Read the model definition and answer for the solid it produces. Units are mm, in the model's axes. Face numbers are marked on the shaded views. A direction names the side the tool comes from. Round coordinates to 2 decimals unless told otherwise and drop trailing zeros. Write each loop counter-clockwise with the first axis right and the second up, starting at its lowest first coordinate (ties: lowest second). Pieces come first, ordered by that corner, then holes. Notation, with made-up numbers: (31.25, 76.25) - (80.25, 76.25) arc R7 cw to (80.25, 82.25) - close; hole circle Ø8 at (10.25, -12.75). An arc over 180 degrees is marked (long way). Use one line per item in the form item = value. Start each with the question number.
1) Each of these flat-tipped pins is pushed along its axis until it touches: pin 1 (3 mm diameter, centred on x = 5.5, z = 3.5, fed in from -Y); pin 2 (1 mm diameter, centred on x = 8, z = 7.5, fed in from +Y); pin 3 (2 mm diameter, centred on x = 3.5, z = 4, fed in from -Y); pin 4 (2 mm diameter, centred on x = -21, z = -14.5, fed in from +Y). Where does it stop, or does it pass through?
2) The part is cut by section D-D, the plane x = -22.5. Give the vertices of the cut face in (y, z), plus the area to 3 significant figures.
3) The part is cut by section A-A, the plane x = -7.5. Give the vertices of the cut face in (y, z), plus the area to 3 significant figures.
4) For a pull along X with two mould halves and no side action, classify the marked faces 1, 2 and 3 as released by +X, released by -X, zero draft, split by the parting line, or undercut.
5) The part is cut by section B-B, the plane y = -1.5. Give the vertices of the cut face in (x, z).
6) The part is cut by section C-C, the plane z = 6. Give the vertices of the cut face in (x, y), plus the area to 3 significant figures.
7) Consider line 1 along X through (y, z) = (2.5, -17); line 2 along Z through (x, y) = (-17, -2.75); line 3 along Z through (x, y) = (-14, -0.75). Determine where each line is inside the solid, lowest interval first. Write a range as from..to.
8) For the marked faces 4, 5, 6, 7 and 8, determine the directions among +Z, -Z, +X, -X, +Y, -Y from which every point of the face is accessible in a straight line to the end or side of a thin tool.
from build123d import *

# Parameters (mm, degrees)
SKETCH_1_W          = 35
SKETCH_1_H          = 32
EXTRUDE_1_DEPTH     = 2
CUT_EXTRUDE_2_DEPTH = 2
SKETCH_3_W          = 35
SKETCH_3_H          = 4
EXTRUDE_2_DEPTH     = 4
SKETCH_4_W          = 35
SKETCH_4_H          = 2
CUT_EXTRUDE_3_DEPTH = 2
SKETCH_5_W          = 35
SKETCH_5_H          = 2
CUT_EXTRUDE_4_DEPTH = 2
SKETCH_6_W          = 5
SKETCH_6_H          = 4.571428571
SKETCH_6_H_2        = 4.571428572
EXTRUDE_3_DEPTH     = 2
SKETCH_7_W          = 25
SKETCH_7_H          = 4.571428572
SKETCH_7_H_2        = 4.571428571
CUT_EXTRUDE_5_DEPTH = 1
SKETCH_9_R          = 1
EXTRUDE_4_DEPTH     = 28
EXTRUDE_START       = -5
SKETCH_9_3_R        = 1
EXTRUDE_5_DEPTH     = 35


with BuildPart() as part:
    # 草图1 → 凸台-拉伸1 (new body)
    with BuildSketch(Plane(origin=(0, 0, 0), x_dir=(1, 0, 0), z_dir=(0, 1, 0))):
        with Locations((-7.669902913, 4.366504854)):
            Rectangle(SKETCH_1_W, SKETCH_1_H)
    extrude(amount=EXTRUDE_1_DEPTH)

    # 草图1<3> → 切除-拉伸2 (cut)
    with BuildSketch(Plane(origin=(0, 0, 0), x_dir=(1, 0, 0), z_dir=(0, 1, 0))):
        Polygon((-7.669902913, 4.366504854), (-20.169902913, 15.795076283), (-20.169902913, -7.062066574), align=None)
        Polygon((4.830097087, 15.795076283), (-20.169902913, 15.795076283), (-7.669902913, 4.366504854), align=None)
        Polygon((4.830097087, 15.795076283), (-7.669902913, 4.366504854), (4.830097087, -7.062066574), align=None)
        Polygon((4.830097087, -7.062066574), (-7.669902913, 4.366504854), (-20.169902913, -7.062066574), align=None)
    extrude(amount=CUT_EXTRUDE_2_DEPTH, mode=Mode.SUBTRACT)

    # 草图3 → 凸台-拉伸2 (add)
    with BuildSketch(Plane.XZ):
        with Locations((-7.669902913, -18.366504854)):
            Rectangle(SKETCH_3_W, SKETCH_3_H)
        with Locations((-7.669902913, 9.633495146)):
            Rectangle(SKETCH_3_W, SKETCH_3_H)
    extrude(amount=EXTRUDE_2_DEPTH)

    # 草图4 → 切除-拉伸3 (cut)
    with BuildSketch(Plane(origin=(0, 0, 7.633495146), x_dir=(-1, 0, 0), z_dir=(0, 0, -1))):
        with Locations((7.669902913, -1)):
            Rectangle(SKETCH_4_W, SKETCH_4_H)
    extrude(amount=-CUT_EXTRUDE_3_DEPTH, mode=Mode.SUBTRACT)

    # 草图5 → 切除-拉伸4 (cut)
    with BuildSketch(Plane.XY.offset(-16.366504854)):
        with Locations((-7.669902913, -1)):
            Rectangle(SKETCH_5_W, SKETCH_5_H)
    extrude(amount=-CUT_EXTRUDE_4_DEPTH, mode=Mode.SUBTRACT)

    # 草图6 → 凸台-拉伸3 (add)
    with BuildSketch(Plane(origin=(0, 2, 0), x_dir=(1, 0, 0), z_dir=(0, 1, 0))):
        with Locations((7.330097087, 18.080790568)):
            Rectangle(SKETCH_6_W, SKETCH_6_H)
        with Locations((7.330097087, -9.34778086)):
            Rectangle(SKETCH_6_W, SKETCH_6_H_2)
        with Locations((-22.669902913, -9.34778086)):
            Rectangle(SKETCH_6_W, SKETCH_6_H_2)
        with Locations((-22.669902913, 18.080790568)):
            Rectangle(SKETCH_6_W, SKETCH_6_H)
    extrude(amount=EXTRUDE_3_DEPTH)

    # 草图7 → 切除-拉伸5 (cut)
    with BuildSketch(Plane(origin=(0, 2, 0), x_dir=(1, 0, 0), z_dir=(0, 1, 0))):
        with Locations((-7.669902913, -9.34778086)):
            Rectangle(SKETCH_7_W, SKETCH_7_H)
        with Locations((-7.669902913, 18.080790568)):
            Rectangle(SKETCH_7_W, SKETCH_7_H_2)
    extrude(amount=-CUT_EXTRUDE_5_DEPTH, mode=Mode.SUBTRACT)

    # 草图9 → 凸台-拉伸4 (add)
    with BuildSketch(Plane(origin=(-20.169902913, 0, 0), x_dir=(0, 0, -1), z_dir=(1, 0, 0))):
        with BuildLine():
            Line((17.080790569, 4), (19.080790569, 4))
            ThreePointArc((19.080790569, 4), (18.080790569, 5), (17.080790569, 4))
        make_face()
        with BuildLine():
            ThreePointArc((17.080790569, 4), (18.080790569, 3), (19.080790569, 4))
            Line((19.080790569, 4), (17.080790569, 4))
        make_face()
        with Locations(Location((-9.34778086, 4, 0), (0, 0, 180))):
            Circle(SKETCH_9_R)
    extrude(amount=EXTRUDE_4_DEPTH)

    # 草图9<3> → 凸台-拉伸5 (add)
    with BuildSketch(Plane(origin=(-20.169902913, 0, 0), x_dir=(0, 0, -1), z_dir=(1, 0, 0)).offset(EXTRUDE_START)):
        with Locations(Location((18.080790569, 4, 0), (0, 0, 180))):
            Circle(SKETCH_9_3_R)
        with Locations(Location((-9.34778086, 4, 0), (0, 0, 180))):
            Circle(SKETCH_9_3_R)
    extrude(amount=EXTRUDE_5_DEPTH)


solid = part.part
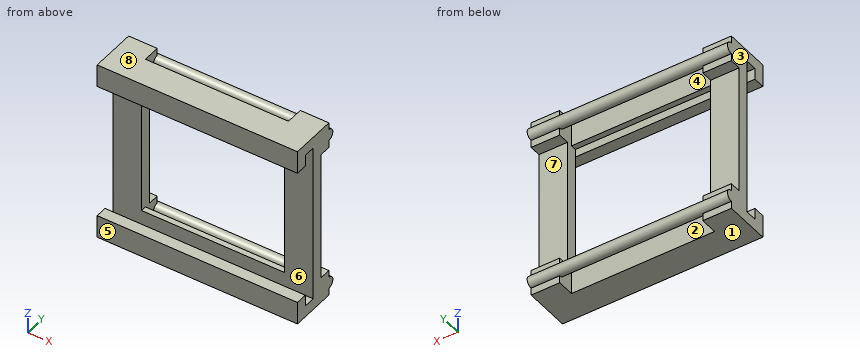
Geometry results:
q1.pin_1 = 0
q1.pin_2 = 4
q1.pin_3 = through
q1.pin_4 = 2
q2.outline = (-4, -20.37) - (4, -20.37) - (4, -19.08) arc R1 ccw to (4, -17.08) - (4, -15.8) - (2, -15.8) - (2, 7.06) - (4, 7.06) - (4, 8.35) arc R1 ccw to (4, 10.35) - (4, 11.63) - (-4, 11.63) - (-4, 7.63) - (-2, 7.63) - (-2, 9.63) - (0, 9.63) - (0, -18.37) - (-2, -18.37) - (-2, -16.37) - (-4, -16.37) - close
q2.area = 109 mm2
q3.outline = (-4, -20.37) - (1, -20.37) - (1, -15.8) - (0, -15.8) - (0, -18.37) - (-2, -18.37) - (-2, -16.37) - (-4, -16.37) - close; (-4, 7.63) - (-2, 7.63) - (-2, 9.63) - (0, 9.63) - (0, 7.06) - (1, 7.06) - (1, 11.63) - (-4, 11.63) - close; circle Ø2 at (4, -18.08); circle Ø2 at (4, 9.35)
q3.area = 39.4 mm2
q4.face_1 = zero draft
q4.face_2 = undercut
q4.face_3 = released by -X
q5.outline = (-25.17, -20.37) - (9.83, -20.37) - (9.83, -18.37) - (-25.17, -18.37) - close; (-25.17, 9.63) - (9.83, 9.63) - (9.83, 11.63) - (-25.17, 11.63) - close
q6.outline = (-25.17, 0) - (-20.17, 0) - (-20.17, 2) - (-25.17, 2) - close; (4.83, 0) - (9.83, 0) - (9.83, 2) - (4.83, 2) - close
q6.area = 20.0 mm2
q7.line_1 = -25.17..-20.17, 4.83..9.83
q7.line_2 = -20.37..-16.37, 7.63..11.63
q7.line_3 = -20.37..-18.37, 9.63..11.63
q8.face_4 = +Z, -Z
q8.face_5 = +Z, -Z, +X, -X, -Y
q8.face_6 = +X, -X
q8.face_7 = +X, -X, +Y
q8.face_8 = +Z, +X, -X, +Y, -Y
